Build history of the part. All positions in model axes, mm. A direction names the side the tool comes from. Give positions to 0.01 mm unless a question says otherwise; leave off trailing zeros. Order: outer loops, then holes, each group sorted by start corner. A loop starts at its lowest first (then second) coordinate and runs counter-clockwise, first axis right, second up. Notation, with made-up numbers: M 13.25,60 L 40.25,60 A18 ccw 40.25,80 Z; hole C 70,60 d8. An arc over 180 degrees is marked long. Use CSV: the item, a comma, the result in double quotes. Start each with the question number.
Item 1: Which spindle directions (+Z, -Z, +X, -X, +Y, -Y) get a long thin tool onto all of the face, cutting with end or side? Do faces 1 (the flat face through (-26.5, 7, 0)), 2 (the flat face through (29, 10, -9)), 3 (the cylindrical face through (-28.72, 20.58, 11.39)), 4 (the flat face through (-31, 7, 1)), 5 (the cylindrical face through (-28.78, 17.78, 3.27)). Say none if no direction does.
Item 2: Two-plate mould, pull along Y, no slides. Class faces 6 (the cylindrical face through (28.719, 15.966, 3.521)), 7 (the flat face through (-6.75, 0, -43)), 8 (the flat face through (-28.213, 5.927, -13.93)): pulls with the +Y half, pulls with the -Y half, needs draft (parallel to the pull), parting line crosses it, or undercut.
Item 3: Wall check: line 1 along X through (y, z) = (5.5, -8.5); line 2 along X through (y, z) = (1.2, -43.5) (3 decimals); line 3 along X through (y, z) = (12, 9.5). Give the ranges that are in metal, low to high.
Item 4: Band-saw the part on B-B on z = -18. Write the cut outline in (x, y), plus the area to 3 significant figures.
Item 5: Band-saw the part on C-C on x = -9.25. Write the cut outline in (y, z) (3 decimals).
Item 6: Band-saw the part on D-D on y = 0.75. Write the cut outline in (x, z) (3 decimals).
Item 7: Band-saw the part on A-A on y = 14.75. Write the cut outline in (x, z).
Item 8: Pin check, flat tips, straight feed: P1, Ø7, axis at y = 12, z = 3, coming from the +X side; P2, Ø6.5, axis at x = -1, y = -0.5, coming from the +Z side; P3, Ø6, axis at y = 2, z = -31.5, coming from the -X side; P4, Ø2, axis at y = 12, z = 10, coming from the -X side. Stop position of each tip, or through.
from build123d import *

# Parameters (mm, degrees)
BOSS_EXTRUDE1_DEPTH      = 3
BOSS_EXTRUDE1_DEPTH_BACK = 3
SKETCH1_R                = 1.375
SKETCH1_W                = 23
SKETCH1_H                = 12
SKETCH2_W                = 4.5
SKETCH2_H                = 24
BOSS_EXTRUDE2_DEPTH      = 21
CUT_EXTRUDE3_START       = -4.5
CUT_EXTRUDE3_OUTLINE_R   = 1.25
CUT_EXTRUDE3_DEPTH       = 4.5
CUT_EXTRUDE4_DEPTH       = 82.155714525
CUT_EXTRUDE4_DEPTH_BACK  = 82.155714525
SKETCH8_R                = 4
FILLET1_R                = 12
CHAMFER2_SIZE            = 10
CHAMFER2_SIZE2           = 5.773502692
CHAMFER3_SIZE            = 15
CHAMFER3_SIZE2           = 10
FILLET2_R                = 5


# Read off the part's stored shape, not the designer's step: Cut-Extrude3
with BuildPart() as part:
    # Sketch1 → Boss-Extrude1 (new, two sides: drawn at the far end of the back side and taken through both)
    with BuildSketch(Plane(origin=(0, 0, 0), x_dir=(1, 0, 0), z_dir=(0, 1, 0)).offset(-BOSS_EXTRUDE1_DEPTH_BACK)):
        Polygon((-31, 13.829866561), (-31, -15), (-26.5, -15), (-26.5, 15), (-20.736331389, 35), (20.736331389, 35), (26.5, 15), (26.5, -15), (31, -15), (31, 13.829866561), (20, 52), (-20, 52), align=None)
        with Locations(Location((18.75, 43.5, 0), (0, 0, 270))):
            Circle(SKETCH1_R, mode=Mode.SUBTRACT)
        with Locations(Location((-9.25, 43.5, 0), (0, 0, 270))):
            Circle(SKETCH1_R, mode=Mode.SUBTRACT)
        with Locations((4.75, 43.5)):
            Rectangle(SKETCH1_W, SKETCH1_H, mode=Mode.SUBTRACT)
    extrude(amount=BOSS_EXTRUDE1_DEPTH + BOSS_EXTRUDE1_DEPTH_BACK)

    # Sketch2 → Boss-Extrude2 (add)
    with BuildSketch(Plane(origin=(0, 3, 0), x_dir=(1, 0, 0), z_dir=(0, 1, 0))):
        with Locations((-28.75, -3)):
            Rectangle(SKETCH2_W, SKETCH2_H)
        with Locations((28.75, -3)):
            Rectangle(SKETCH2_W, SKETCH2_H)
    extrude(amount=BOSS_EXTRUDE2_DEPTH)

    # Cut-Extrude3 outline → Cut-Extrude3 (cut)
    with BuildSketch(Plane(origin=(-26.5, 0, 0), x_dir=(0, 0, -1), z_dir=(1, 0, 0)).offset(CUT_EXTRUDE3_START)):
        with Locations((-3, 19)):
            Circle(CUT_EXTRUDE3_OUTLINE_R)
        with Locations((4, 12)):
            Circle(CUT_EXTRUDE3_OUTLINE_R)
        with Locations((-3, 5)):
            Circle(CUT_EXTRUDE3_OUTLINE_R)
        with Locations((-10, 12)):
            Circle(CUT_EXTRUDE3_OUTLINE_R)
    extrude(amount=CUT_EXTRUDE3_DEPTH, mode=Mode.SUBTRACT)

    # Sketch8 → Cut-Extrude4 (cut, two sides: drawn at the far end of the back side and taken through both)
    with BuildSketch(Plane(origin=(-26.5, 0, 0), x_dir=(0, 0, -1), z_dir=(1, 0, 0)).offset(-CUT_EXTRUDE4_DEPTH_BACK)):
        with Locations((-3, 12)):
            Circle(SKETCH8_R)
    extrude(amount=CUT_EXTRUDE4_DEPTH + CUT_EXTRUDE4_DEPTH_BACK, mode=Mode.SUBTRACT)

    # Fillet1
    fillet1_edges = [part.edges().sort_by_distance(p)[0] for p in [
        (28.75, -3, 15),
        (-28.75, -3, 15),
        (-28.75, 24, -9),
        (28.75, 24, -9),
        (28.75, 24, 15),
        (-28.75, 24, 15),
    ]]
    fillet(fillet1_edges, radius=FILLET1_R - 0.0001)  # a hair under: the kernel refuses the full size

    # Chamfer2
    chamfer2_edges = [part.edges().sort_by_distance(p)[0] for p in [
        (-28.75, 3, -9),
        (28.75, 3, -9),
    ]]
    chamfer2_side = [part.faces().sort_by_distance(p)[0] for p in [
        (-1.966040558, 3, -36.302482854),
    ]]
    chamfer(chamfer2_edges, length=CHAMFER2_SIZE, length2=CHAMFER2_SIZE2, reference=chamfer2_side[0])

    # Chamfer3
    chamfer3_edges = [part.edges().sort_by_distance(p)[0] for p in [
        (-20, 0, -52),
    ]]
    chamfer3_side = [part.faces().sort_by_distance(p)[0] for p in [
        (-25.663082519, 0.130215421, -32.349034961),
    ]]
    chamfer(chamfer3_edges, length=CHAMFER3_SIZE, length2=CHAMFER3_SIZE2, reference=chamfer3_side[0])

    # Fillet2
    fillet2_edges = [part.edges().sort_by_distance(p)[0] for p in [
        (20, 0, -52),
        (-10, 0, -52),
    ]]
    fillet(fillet2_edges, radius=FILLET2_R)


solid = part.part
Model answer:
1,face 1,"+Z, +Y, -Y"
1,face 2,"-Z, +X, -X, +Y"
1,face 3,"+Z, +X, -X, +Y"
1,face 4,"+Z, -Z, -X, +Y, -Y"
1,face 5,"-X"
2,face 6,"undercut"
2,face 7,"needs draft"
2,face 8,"pulls with the +Y half"
3,line 1,"x = -31 to -26.5, 26.5 to 31"
3,line 2,"x = -18.347 to -10.625, -7.875 to -6.75, 16.25 to 17.375, 20.125 to 22.45"
3,line 3,"x = 26.5 to 31"
4,outline,"M -29.8,-3 L -25.64,-3 L -25.64,3.58 L -29.8,3.58 Z; M 25.64,-3 L 29.8,-3 L 29.8,3.58 L 25.64,3.58 Z"
4,area,"54.8 mm^2"
5,outline,"M -3,-51.815 L 3,-51.815 L 3,-44.875 L -3,-44.875 Z; M -3,-42.125 L 3,-42.125 L 3,-35 L -3,-35 Z"
6,outline,"M -31,-13.83 L -24.154,-37.587 L -11.47,-50.503 A5 ccw -7.902,-52 L 16.237,-52 A5 ccw 21.042,-48.385 L 31,-13.83 L 31,11.714 L 26.5,11.714 L 26.5,-15 L 20.736,-35 L -20.736,-35 L -26.5,-15 L -26.5,11.714 L -31,11.714 Z; hole C -9.25,-43.5 d2.75; hole M -6.75,-49.5 L 16.25,-49.5 L 16.25,-37.5 L -6.75,-37.5 Z; hole C 18.75,-43.5 d2.75"
7,outline,"M -31,-8.68 L -26.5,-8.68 L -26.5,0.1 L -31,0.1 Z; M -31,5.9 L -26.5,5.9 L -26.5,14.68 L -31,14.68 Z; M 26.5,-8.68 L 31,-8.68 L 31,0.1 L 26.5,0.1 Z; M 26.5,5.9 L 31,5.9 L 31,14.68 L 26.5,14.68 Z"
8,P1,"passes through"
8,P2,"stops at z = -35"
8,P3,"stops at x = -26.77"
8,P4,"stops at x = 26.5"
